Source: three-view drawing plus pictorial views. Frame: mm from the lowest corner of the part. A direction names the side the tool comes from. Round coordinates to 2 decimals unless told otherwise and drop trailing zeros. Loops run counter-clockwise (first coordinate to the right, second up) from the corner with the lowest first, then second, coordinate; pieces in that order, holes last. Notation, with made-up numbers: (68.25, 42.25) -> (112.25, 42.25) arc R23 ccw to (112.25, 57.25) -> close; hole circle Ø7 at (-13.75, -34). An arc over 180 degrees is marked (long way). Answer in a Markdown table with one row per item. Add a question column.
Q1. Ray query, L1, parallel to Y at x = 36.5, z = 26.75; L2, parallel to X at y = 39, z = 24.75; L3, parallel to X at y = 6.5, z = 17.75. Return the intervals inside material, ascending. Write a range as from..to.
Q2. Section C-C, the plane z = 17.25. Output: boundary loops of the cut face in (x, y) (1 decimal), and give its area (3 significant figures).
Q3. Pin query (flat end, axial travel): pin 1 (2 mm diameter, centred on x = 1, y = 12.5, fed in from -Z); pin 2 (12 mm diameter, centred on x = 20.5, y = 12, fed in from +Z); pin 3 (2 mm diameter, centred on y = 27, z = 11, fed in from -X); pin 4 (5.5 mm diameter, centred on x = 50.5, z = 11.5, fed in from -Y). Return the tip coordinate at first contact, or that it passes through.
Q4. Section B-B, the plane y = 17. Output: boundary loops of the cut face in (x, z).
Q5. Mould query, pull axis Y, two halves, no side actions, for the marked faces 1, 2 and 3. Classes: pulls with the +Y half, pulls with the -Y half, needs draft (parallel to the pull), parting line crosses it, or undercut.
Q6. Section D-D, the plane z = 22.5. Output: boundary loops of the cut face in (x, y) (1 decimal).
Q7. Section A-A, the plane x = 5. Output: boundary loops of the cut face in (y, z), and give its area (3 significant figures).
Q8. Reachability of the marked faces 4 and 5 from +Z, -Z, +X, -X, +Y, -Y: full face, straight path, thin tool, end or side. Return the list, or none.
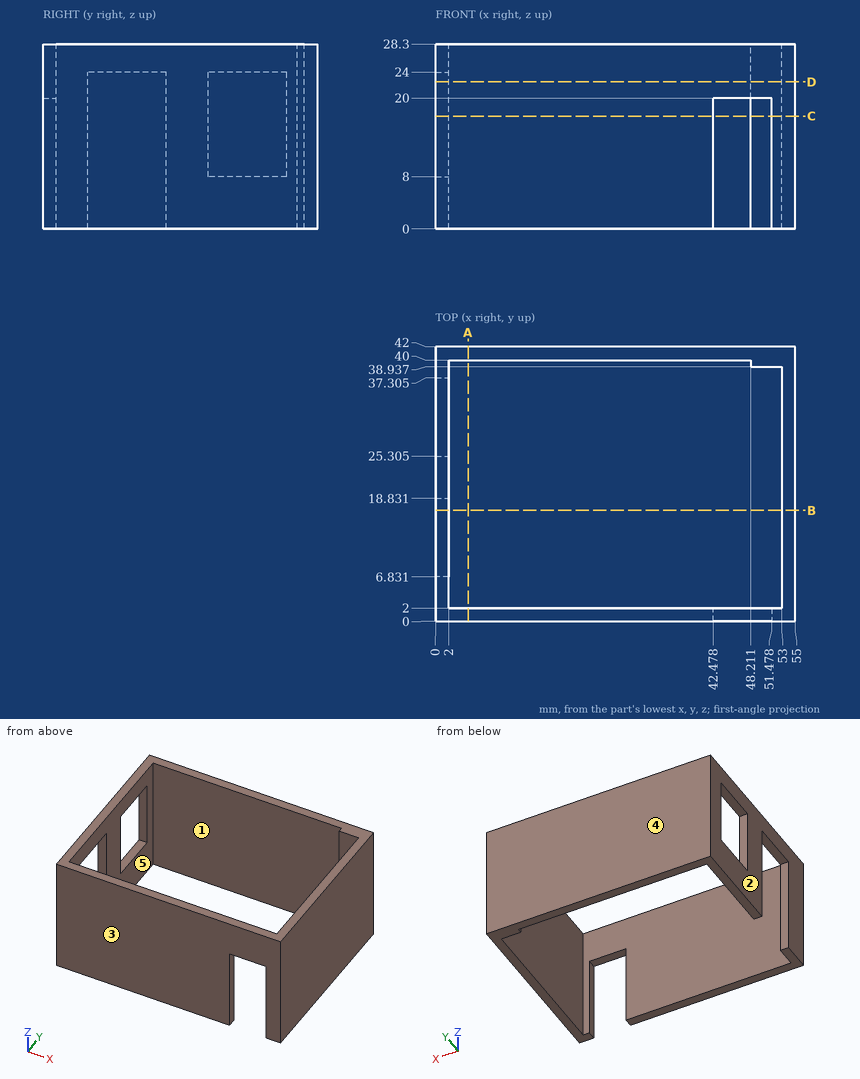
Answer block:
| question | item | result |
|---|---|---|
| 1 | L1 | 0..2, 40..42 |
| 1 | L2 | 0..2, 48.21..55 |
| 1 | L3 | 0..2, 53..55 |
| 2 | outline | (0, 0) -> (42.5, 0) -> (42.5, 2) -> (2, 2) -> (2, 6.8) -> (0, 6.8) -> close; (0, 18.8) -> (2, 18.8) -> (2, 25.3) -> (0, 25.3) -> close; (0, 37.3) -> (2, 37.3) -> (2, 40) -> (48.2, 40) -> (48.2, 38.9) -> (53, 38.9) -> (53, 2) -> (51.5, 2) -> (51.5, 0) -> (55, 0) -> (55, 42) -> (0, 42) -> close |
| 2 | area | 311 mm^2 |
| 3 | pin 1 | z = 24 |
| 3 | pin 2 | through |
| 3 | pin 3 | x = 53 |
| 3 | pin 4 | y = 0 |
| 4 | outline | (0, 24) -> (2, 24) -> (2, 28.3) -> (0, 28.3) -> close; (53, 0) -> (55, 0) -> (55, 28.3) -> (53, 28.3) -> close |
| 5 | face 1 | undercut |
| 5 | face 2 | needs draft |
| 5 | face 3 | pulls with the -Y half |
| 6 | outline | (0, 0) -> (55, 0) -> (55, 42) -> (0, 42) -> (0, 37.3) -> (2, 37.3) -> (2, 40) -> (48.2, 40) -> (48.2, 38.9) -> (53, 38.9) -> (53, 2) -> (2, 2) -> (2, 6.8) -> (0, 6.8) -> close; (0, 18.8) -> (2, 18.8) -> (2, 25.3) -> (0, 25.3) -> close |
| 7 | outline | (0, 0) -> (2, 0) -> (2, 28.3) -> (0, 28.3) -> close; (40, 0) -> (42, 0) -> (42, 28.3) -> (40, 28.3) -> close |
| 7 | area | 113 mm^2 |
| 8 | face 4 | +Z, -Z, +X, -X, +Y |
| 8 | face 5 | +Z, -Z |
